The model under review builds one solid part; all positions refer to its coordinate system, in mm. Face numbers are marked on the shaded views. Give positions to 0.01 mm unless a question says otherwise; leave off trailing zeros. Order: outer loops, then holes, each group sorted by start corner. A loop starts at its lowest first (then second) coordinate and runs counter-clockwise, first axis right, second up. Notation, with made-up numbers: (81.25, -33.75) - (104.25, -33.75) arc R13 cw to (104.25, -29.75) - close; hole circle Ø5 at (6.5, 16). An arc over 180 degrees is marked (long way). Write item = value, one per line. Start each with the question number.
1. Mouldability with a two-part tool opening along Y and no side actions: class the marked faces 1 and 2 as pulls with the +Y half, pulls with the -Y half, needs draft (parallel to the pull), parting line crosses it, or undercut.
2. For P1, Ø1.5, axis at x = 29, z = 6.5, coming from the +Y side; P2, Ø10, axis at x = -50, z = 0, coming from the -Y side; P3, Ø2, axis at y = 57.5, z = 52, coming from the -X side; P4, Ø5, axis at x = 60.5, z = 20, coming from the -Y side, all flat-tipped, find the tip position at first contact; note any pin that passes through.
3. We need section D-D, the plane y = 0. Give the boundary of the cut face in (x, z).
4. We need section B-B, the plane z = 51.5. State how many separate pieces and enclosed holes the cut face has, and give its area (3 significant figures).
5. We need section C-C, the plane y = 17.5. Give the boundary of the cut face in (x, z).
6. Wall thickness on probe 1 along Z at (x, y) = (-47, -15.5); probe 2 along X at (y, z) = (-36, 8); probe 3 along Y at (x, z) = (63.5, 38.5): over which ranges is each line inside the solid? List them lowest first.
7. We need section A-A, the plane x = 0. Give the boundary of the cut face in (y, z), and give its area (3 significant figures).
from build123d import *

# Parameters (mm, degrees)
F1_START        = -67.31
F0_R            = 78.74
F1_DEPTH        = 6.858
F2_R            = 2.285444595
F3_DEPTH        = 139.7
F3_COPIES_COUNT = 18


# Not quite as in the source:
# - a pattern or mirror of a feature is missing from the dataset's text; its kind, count and spacing are read off the source's solid


with BuildPart() as f1:
    # F0 (on Top) → F1 (new body)
    with BuildSketch(Plane.XY.offset(F1_START)):
        Circle(F0_R)
    extrude(amount=-F1_DEPTH)

    # F2 (on face) → F3 (join)
    with BuildSketch(Plane.XY.offset(-67.31)):
        with Locations((0, 74.8899579048)):
            Circle(F2_R)
    f3 = extrude(amount=F3_DEPTH)

    # F3_copies: F3 ×18 about axis
    f3_copies_axis = Axis((0, 0, 0), (0, 0, 1))
    for i in range(1, F3_COPIES_COUNT):
        add(f3.rotate(f3_copies_axis, i * 360 / F3_COPIES_COUNT))


solid = f1.part
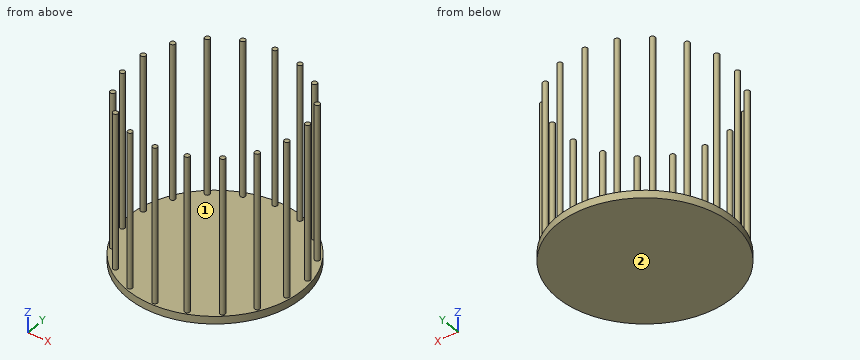
Model answer:
q1.face_1 = undercut
q1.face_2 = needs draft
q2.P1 = through
q2.P2 = -59.65
q2.P3 = -50.42
q2.P4 = -38.78
q3.outline = (-78.74, -74.17) - (78.74, -74.17) - (78.74, -67.31) - (-78.74, -67.31) - close
q4.separate_pieces = 18
q4.enclosed_holes = 0
q4.area = 295 mm2
q5.outline = (-76.77, -74.17) - (76.77, -74.17) - (76.77, -67.31) - (-76.77, -67.31) - close
q6.probe_1 = -74.17 to -67.31
q6.probe_2 = -66.63 to -63.09, 63.09 to 66.63
q6.probe_3 = -39.28 to -35.61, 35.61 to 39.28
q7.outline = (-78.74, -74.17) - (78.74, -74.17) - (78.74, -67.31) - (77.18, -67.31) - (77.18, 72.39) - (72.6, 72.39) - (72.6, -67.31) - (-72.6, -67.31) - (-72.6, 72.39) - (-77.18, 72.39) - (-77.18, -67.31) - (-78.74, -67.31) - close
q7.area = 2,360 mm2
